The listing builds one solid part. Answer for the finished solid, in the listing's coordinates (mm). Round coordinates to 2 decimals unless told otherwise and drop trailing zeros. Write each loop counter-clockwise with the first axis right and the second up, starting at its lowest first coordinate (ties: lowest second). Pieces come first, ordered by that corner, then holes. Notation, with made-up numbers: M 35,72 L 94,72 A19 cw 94,103 Z; hole C 11,87.5 d2. An arc over 180 degrees is marked long. Put each result on its own line as item: value. Start each with the question number.
```python
from build123d import *

# Parameters (mm, degrees)
SKETCH1_R           = 4
SKETCH1_R_2         = 4.15
BOSS_EXTRUDE2_DEPTH = 5


with BuildPart() as part:
    # Sketch1 → Boss-Extrude2 (new body)
    # profile 1 of 2: a face of its own
    with BuildSketch(Plane.XY):
        with BuildLine():
            Line((-25, -20.3), (25, -20.3))
            ThreePointArc((25, -20.3), (28.288479467, -21.007133431), (30.995610492, -23.003524301))
            Line((30.995610492, -23.003524301), (5.995610492, 5.296475699))
            ThreePointArc((5.995610492, 5.296475699), (0, 8), (-5.995610492, 5.296475699))
            Line((-5.995610492, 5.296475699), (-30.995610492, -23.003524301))
            ThreePointArc((-30.995610492, -23.003524301), (-28.288479467, -21.007133431), (-25, -20.3))
        make_face()
        Circle(SKETCH1_R, mode=Mode.SUBTRACT)
    # profile 2 of 2: a face of its own
    with BuildSketch(Plane.XY):
        with BuildLine():
            ThreePointArc((25, -20.3), (28.288479467, -21.007133431), (30.995610492, -23.003524301))
            ThreePointArc((30.995610492, -23.003524301), (32.292866569, -31.588479467), (25, -36.3))
            Line((25, -36.3), (-25, -36.3))
            ThreePointArc((-25, -36.3), (-32.292866569, -31.588479467), (-30.995610492, -23.003524301))
            ThreePointArc((-30.995610492, -23.003524301), (-28.288479467, -21.007133431), (-25, -20.3))
            Line((-25, -20.3), (25, -20.3))
        make_face()
        with Locations((-25, -28.3)):
            Circle(SKETCH1_R_2, mode=Mode.SUBTRACT)
        with Locations((25, -28.3)):
            Circle(SKETCH1_R_2, mode=Mode.SUBTRACT)
    extrude(amount=-BOSS_EXTRUDE2_DEPTH)


solid = part.part
```
Item 1: Section B-B (x = 0) is taken. Give the vertices of the cut face in (y, z), and give its area (4 significant figures).
Item 2: Section C-C (y = 1.5) is taken. Give the vertices of the cut face in (x, z), and give its area (3 significant figures).
Item 3: Section A-A (y = -28.3) is taken. Give the vertices of the cut face in (x, z).
Item 4: Section D-D (z = -3.45) is taken. Give the vertices of the cut face in (x, y), and give its area (3 significant figures).
Item 5: Consider line 1 along X through (y, z) = (-32, -3.7); line 2 along Y through (x, z) = (0, -3.45); line 3 along Y through (x, z) = (-2, -2.45). Determine where each line is inside the solid, lowest interval first. Write a range as [from, to].
Item 6: Determine the mould class of faces 1 (the flat face through (0, -19, 0)), 2 (the cylindrical face through (0, 8, -2)), 3 (the cylindrical face through (-0.867, -3.905, -2.465)) for opening direction Y: released by +Y, released by -Y, zero draft, split by the parting line, or undercut.
Item 7: Flat-ended cylindrical pins translate along their axes: pin 1 (5 mm diameter, centred on x = -25, y = -28.3, fed in from -Z); pin 2 (3 mm diameter, centred on x = 15, z = -3.5, fed in from +Y); pin 3 (3 mm diameter, centred on x = -13.5, z = -2, fed in from +Y). Find the tip coordinate at first contact, or state that the pin passes through.
Output values:
1. outline: M -36.3,-5 L -4,-5 L -4,0 L -36.3,0 Z; M 4,-5 L 8,-5 L 8,0 L 4,0 Z
1. area: 181.5 mm^2
2. outline: M -9.35,-5 L -3.71,-5 L -3.71,0 L -9.35,0 Z; M 3.71,-5 L 9.35,-5 L 9.35,0 L 3.71,0 Z
2. area: 56.4 mm^2
3. outline: M -33,-5 L -29.15,-5 L -29.15,0 L -33,0 Z; M -20.85,-5 L 20.85,-5 L 20.85,0 L -20.85,0 Z; M 29.15,-5 L 33,-5 L 33,0 L 29.15,0 Z
4. outline: M -31,-23 A8 ccw -25,-36.3 L 25,-36.3 A8 ccw 31,-23 L 6,5.3 A8 ccw -6,5.3 Z; hole C -25,-28.3 d8.3; hole C 0,0 d8; hole C 25,-28.3 d8.3
4. area: 1,750 mm^2
5. line 1: x = [-32.09, -26.88], [-23.12, 23.12], [26.88, 32.09]
5. line 2: y = [-36.3, -4], [4, 8]
5. line 3: y = [-36.3, -3.46], [3.46, 7.75]
6. face 1: zero draft
6. face 2: released by +Y
6. face 3: undercut
7. pin 1: passes through
7. pin 2: stops at y = -3.2
7. pin 3: stops at y = -1.5
